Here's how the part is built. I have some questions about the finished solid (model axes, mm). Give positions to 0.01 mm unless a question says otherwise; leave off trailing zeros. Write each loop counter-clockwise with the first axis right and the second up, starting at its lowest first coordinate (ties: lowest second). Pieces come first, ordered by that corner, then holes. Notation, with made-up numbers: (37, 5) -> (82, 5) arc R25 ccw to (82, 19) -> close; hole circle Ø3 at (3, 46). An arc over 180 degrees is marked (long way). Put each result on its own line as item: value. Start each with the question number.
from build123d import *

# Parameters (mm, degrees)
F0_W     = 25.4
F0_H     = 25.4
F2_R     = 12.69999
F3_R     = 10
F4_DEPTH = 20.32
F5_R     = 10


# Not quite as in the source:
# - a fillet or chamfer is up to 0.001 mm smaller than in the source, because OpenCascade refuses the exact size


with BuildPart() as f1:
    # F0 (on Front) → F1 (revolve)
    with BuildSketch(Plane.XZ):
        with Locations((12.7, 12.7)):
            Rectangle(F0_W, F0_H)
    revolve(axis=Axis((0, 0, 17.3243917525), (0, 0, 1)))

    # F2 (radius 12.7 in the source; OpenCascade refuses exactly that, so slightly less here)
    f2_edges = [f1.edges().sort_by_distance(p)[0] for p in [
        (-25.4, 0, 0),
        (-25.4, 0, 25.4),
        (25.4, 0, 12.7),
    ]]
    fillet(f2_edges, radius=F2_R)

    # F3 (on face) → F4 (cut)
    with BuildSketch(Plane.XY.offset(25.4)):
        Circle(F3_R)
    extrude(amount=-F4_DEPTH, mode=Mode.SUBTRACT)

    # F5
    f5_edges = [f1.edges().sort_by_distance(p)[0] for p in [
        (-10, 0, 5.08),
    ]]
    fillet(f5_edges, radius=F5_R)


solid = f1.part
1) Thinking about a two-plate mould opening in Y: for faces 1 (the cylindrical face through (-2.17, -9.76, 20.31)), 2 (the flat face through (0.1, -10.3, 25.4)), which applies, released by +Y, released by -Y, zero draft, split by the parting line, or undercut?
2) I want a section at D-D, the plane z = 9. Write out the boundary of the cut face in (x, y).
3) I'm going to push flat-ended pins straight in: pin 1 Ø1 at (x, y) = (-13.5, 12.5) entering from +Z; pin 2 Ø8 at (x, z) = (16.5, 23) entering from -Y; pin 3 Ø5 at (y, z) = (13.5, 9.5) entering from -X. Where does each tip first touch, or does it pass through?
4) I want a section at C-C, the plane z = 21.25. Write out the boundary of the cut face in (x, y), and give its area (3 significant figures).
5) I need wall thicknesses on probe 1 along Y at (x, z) = (6, 11.75); probe 2 along Y at (x, z) = (-5, 10); probe 3 along Z at (x, y) = (11, -7.5). Which ranges of each line are inside material? Lowest first, please.
Established:
1. face 1: undercut
1. face 2: zero draft
2. outline: circle Ø49.7 at (0, 0); hole circle Ø15.88 at (0, 0)
3. pin 1: stops at z = 24.29
3. pin 2: stops at y = -18.48
3. pin 3: stops at x = -22.58
4. outline: circle Ø44.18 at (0, 0); hole circle Ø20 at (0, 0)
4. area: 1,220 mm2
5. probe 1: y = -24.64 to -7.27, 7.27 to 24.64
5. probe 2: y = -24.61 to -7.01, 7.01 to 24.61
5. probe 3: z = 0.01 to 25.39
